```python
from build123d import *

# Parameters (mm, degrees)
SKETCH1_R           = 1.737885662
SKETCH1_R_2         = 1.873200063
SKETCH1_R_3         = 1.690089146
SKETCH1_R_4         = 1.754205974
SKETCH1_R_5         = 1.7
SKETCH1_R_6         = 4.5
SKETCH1_R_7         = 9.5
SKETCH1_W           = 3
SKETCH1_H           = 10
SKETCH1_W_2         = 10
SKETCH1_H_2         = 3
BOSS_EXTRUDE1_DEPTH = 3
FILLET1_R           = 10
FILLET2_R           = 3
FILLET3_R           = 2


with BuildPart() as part:
    # Sketch1 → Boss-Extrude1 (new body)
    with BuildSketch(Plane.XY):
        Polygon((147.061964125, -92.970138098), (147.061964125, -71.856515964), (147.061964125, -67.856515964), (175.843347401, -67.856515964), (175.843347401, -87.856515964), (170.198907285, -87.856515964), (170.198907285, -135.887076434), (175.843347401, -135.887076434), (175.843347401, -155.887076434), (147.061964125, -155.887076434), (147.061964125, -151.887076434), (147.061964125, -130.215533927), (127.203791419, -130.215533927), (127.203791419, -111.591712302), (127.203791419, -92.970138098), align=None)
        with Locations((130.520049527, -96.082032258)):
            Circle(SKETCH1_R, mode=Mode.SUBTRACT)
        with Locations((161.520049527, -96.082032258)):
            Circle(SKETCH1_R_2, mode=Mode.SUBTRACT)
        with Locations((130.520049527, -127.114221831)):
            Circle(SKETCH1_R_3, mode=Mode.SUBTRACT)
        with Locations((161.520049527, -127.082032258)):
            Circle(SKETCH1_R_4, mode=Mode.SUBTRACT)
        with Locations((154.157584865, -111.662272701)):
            Circle(SKETCH1_R_5, mode=Mode.SUBTRACT)
        with Locations((145.89014032, -119.788596448)):
            Circle(SKETCH1_R_5, mode=Mode.SUBTRACT)
        with Locations((137.763816574, -111.521151903)):
            Circle(SKETCH1_R_5, mode=Mode.SUBTRACT)
        with Locations((146.031261118, -103.394828157)):
            Circle(SKETCH1_R_5, mode=Mode.SUBTRACT)
        with Locations((145.960700719, -111.591712302)):
            Circle(SKETCH1_R_6, mode=Mode.SUBTRACT)
        with Locations((157.960700719, -81.591712302)):
            Circle(SKETCH1_R_7, mode=Mode.SUBTRACT)
        with Locations((157.960700719, -141.591712302)):
            Circle(SKETCH1_R_7, mode=Mode.SUBTRACT)
        with Locations((131.960700719, -111.591712302)):
            Rectangle(SKETCH1_W, SKETCH1_H, mode=Mode.SUBTRACT)
        with Locations((145.960700719, -97.591712302)):
            Rectangle(SKETCH1_W_2, SKETCH1_H_2, mode=Mode.SUBTRACT)
        with Locations((145.960700719, -125.591712302)):
            Rectangle(SKETCH1_W_2, SKETCH1_H_2, mode=Mode.SUBTRACT)
        with Locations((166.293610901, -111.591712302)):
            Rectangle(SKETCH1_W, SKETCH1_H, mode=Mode.SUBTRACT)
    extrude(amount=BOSS_EXTRUDE1_DEPTH)

    # Fillet1
    fillet1_edges = [part.edges().sort_by_distance(p)[0] for p in [
        (147.061964125, -67.856515964, 1.5),
        (175.843347401, -67.856515964, 1.5),
        (175.843347401, -155.887076434, 1.5),
        (147.061964125, -155.887076434, 1.5),
    ]]
    fillet(fillet1_edges, radius=FILLET1_R)

    # Fillet2
    fillet2_edges = [part.edges().sort_by_distance(p)[0] for p in [
        (147.061964125, -130.215533927, 1.5),
        (127.203791419, -130.215533927, 1.5),
        (127.203791419, -92.970138098, 1.5),
        (147.061964125, -92.970138098, 1.5),
    ]]
    fillet(fillet2_edges, radius=FILLET2_R)

    # Fillet3
    fillet3_edges = [part.edges().sort_by_distance(p)[0] for p in [
        (175.843347401, -87.856515964, 1.5),
        (170.198907285, -87.856515964, 1.5),
        (170.198907285, -135.887076434, 1.5),
        (175.843347401, -135.887076434, 1.5),
    ]]
    fillet(fillet3_edges, radius=FILLET3_R)


solid = part.part
```
Work out the finished part from the listing and answer in its coordinate system (mm). A direction names the side the tool comes from. Round coordinates to 2 decimals unless told otherwise and drop trailing zeros. Write each loop counter-clockwise with the first axis right and the second up, starting at its lowest first coordinate (ties: lowest second). Pieces come first, ordered by that corner, then holes.
1) Flat-ended cylindrical pins translate along their axes: P1, Ø0.9, axis at x = 148.5, z = 2, coming from the +Y side; P2, Ø1.5, axis at y = -112, z = 2, coming from the +X side. Find the tip coordinate at first contact, or state that the pin passes through.
2) A cutting plane is placed at B-B on x = 145.5. Determine the outline of the cut face in (y, z).
3) A cutting plane is placed at C-C on y = -114.5. Determine the outline of the cut face in (x, z).
4) Determine the mould class of faces 1 (the face through (161, -67.857, 1)), 2 (the face through (167.794, -112, 1)), 3 (the face through (175.843, -142, 1)), 4 (the face through (148.38, -107.797, 1.479)) for opening direction Y: pulls with the +Y half, pulls with the -Y half, needs draft (parallel to the pull), parting line crosses it, or undercut.
5) A cutting plane is placed at D-D on y = -80. Determine the outline of the cut face in (x, z) (3 decimals).
6) Consider probe 1 along Y at (x, z) = (158, 2.25); probe 2 along X at (y, z) = (-125, 0.8); probe 3 along X at (y, z) = (-81.5, 1). Determine where each line is inside the solid, lowest interval first.
7) A cutting plane is placed at A-A on y = -139. Determine the outline of the cut face in (x, z).
8) Which of the six approach directions +Z, -Z, +X, -X, +Y, -Y give full straight-line access (tool end or side, diameter ignored) to faces 5 (the face through (146, -124.092, 1)), 6 (the face through (170.199, -112, 1)), 7 (the face through (128.106, -93.826, 1.521))?
Entries:
1. P1: stops at y = -72.01
1. P2: stops at x = 170.2
2. outline: (-130.58, 0) - (-127.09, 0) - (-127.09, 3) - (-130.58, 3) - close; (-124.09, 0) - (-121.44, 0) - (-121.44, 3) - (-124.09, 3) - close; (-118.13, 0) - (-116.07, 0) - (-116.07, 3) - (-118.13, 3) - close; (-107.12, 0) - (-105.01, 0) - (-105.01, 3) - (-107.12, 3) - close; (-101.78, 0) - (-99.09, 0) - (-99.09, 3) - (-101.78, 3) - close; (-96.09, 0) - (-92.6, 0) - (-92.6, 3) - (-96.09, 3) - close
3. outline: (127.2, 0) - (130.46, 0) - (130.46, 3) - (127.2, 3) - close; (133.46, 0) - (142.53, 0) - (142.53, 3) - (133.46, 3) - close; (149.39, 0) - (164.79, 0) - (164.79, 3) - (149.39, 3) - close; (167.79, 0) - (170.2, 0) - (170.2, 3) - (167.79, 3) - close
4. face 1: pulls with the +Y half
4. face 2: undercut
4. face 3: needs draft
4. face 4: undercut
5. outline: (147.062, 0) - (148.595, 0) - (148.595, 3) - (147.062, 3) - close; (167.326, 0) - (175.843, 0) - (175.843, 3) - (167.326, 3) - close
6. probe 1: y = -155.89 to -151.09, -132.09 to -91.09, -72.09 to -67.86
6. probe 2: x = 127.2 to 140.96, 150.96 to 170.2
6. probe 3: x = 147.06 to 148.46, 167.46 to 175.84
7. outline: (147.06, 0) - (148.82, 0) - (148.82, 3) - (147.06, 3) - close; (167.1, 0) - (175.84, 0) - (175.84, 3) - (167.1, 3) - close
8. face 5: +Z, -Z
8. face 6: +Z, -Z, +X
8. face 7: +Z, -Z, -X, +Y
